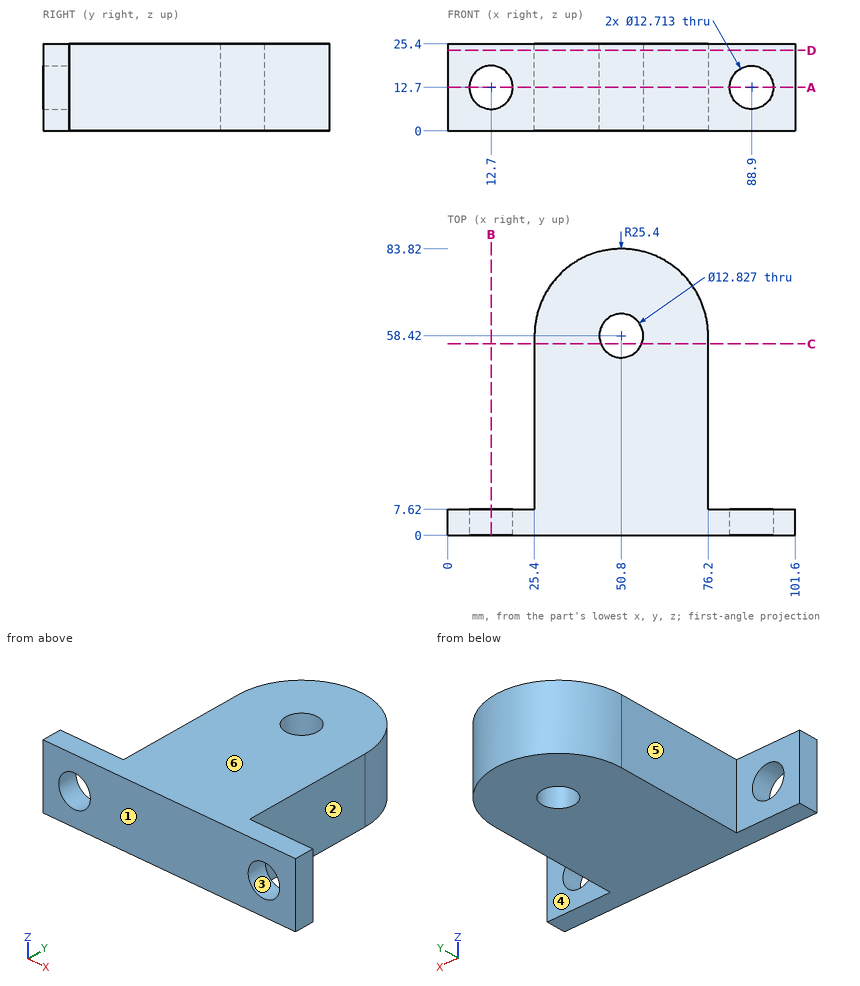
The drawing under review shows one solid part. Ordinate dimensions are in mm from its lowest x, y, z. A direction names the side the tool comes from. Coordinates: 2 decimals unless noted, no trailing zeros. Loops run counter-clockwise (first coordinate to the right, second up) from the corner with the lowest first, then second, coordinate; pieces in that order, holes last. Notation, with made-up numbers: (-33.5, -21.75) - (5.5, -21.75) arc R25 cw to (5.5, -8.75) - close; hole circle Ø7 at (61.5, 43.25). An arc over 180 degrees is marked (long way). Return JSON: item names as keys, results as strings.
Item 1: Take a section at C-C (y = 56). Give the boundary of the cut face in (x, z).
Determined:
{"outline": "(25.4, 0) - (44.86, 0) - (44.86, 25.4) - (25.4, 25.4) - close; (56.74, 0) - (76.2, 0) - (76.2, 25.4) - (56.74, 25.4) - close"}
Item 2: For line 1 (Y direction, x = 50.8, z = 6.75); line 2 (Z direction, x = 88.9, y = 5.5); line 3 (X direction, y = 11.5, z = 10.25), list the stretches that pass through material, from the lowest coordinate up.
Determined:
{"line 1": "y = 0 to 52.01, 64.83 to 83.82", "line 2": "z = 0 to 6.34, 19.06 to 25.4", "line 3": "x = 25.4 to 76.2"}
Item 3: Insertion check: pin 1 (2 mm diameter, centred on y = 71.5, z = 9, fed in from +X); pin 2 (1 mm diameter, centred on y = 74.5, z = 15.5, fed in from -X); pin 3 (16.5 mm diameter, centred on x = 50.8, y = 58.42, fed in from -Z); pin 4 (7.5 mm diameter, centred on x = 92.5, z = 6.5, fed in from +Y). Each pin has a flat end and moves straight along its axis. Give the tip position at first contact, or say it passes through.
Determined:
{"pin 1": "stops at x = 73.14", "pin 2": "stops at x = 30.74", "pin 3": "stops at z = 0", "pin 4": "stops at y = 7.62"}
Item 4: For the marked faces 4, 5 and 6, list the 3-axis set-ups (+Z, -Z, +X, -X, +Y, -Y) from which the entire face can be reached by the end or side of a thin tool; tool diameter is ignored.
Determined:
{"face 4": "+Z, -Z, +X, +Y", "face 5": "+Z, -Z, -X, +Y", "face 6": "+Z, +X, -X, +Y, -Y"}
Item 5: Take a section at B-B (x = 12.7). Give the boundary of the cut face in (y, z).
Determined:
{"outline": "(0, 0) - (7.62, 0) - (7.62, 6.34) - (0, 6.34) - close; (0, 19.06) - (7.62, 19.06) - (7.62, 25.4) - (0, 25.4) - close"}
Item 6: Take a section at A-A (z = 12.7). Give the boundary of the cut face in (x, y), then the cut area to 3 significant figures.
Determined:
{"outline": "(0, 0) - (6.34, 0) - (6.34, 7.62) - (0, 7.62) - close; (19.06, 0) - (82.54, 0) - (82.54, 7.62) - (76.2, 7.62) - (76.2, 58.42) arc R25.4 ccw to (25.4, 58.42) - (25.4, 7.62) - (19.06, 7.62) - close; (95.26, 0) - (101.6, 0) - (101.6, 7.62) - (95.26, 7.62) - close; hole circle Ø12.83 at (50.8, 58.42)", "area": "4,050 mm2"}
Item 7: Take a section at D-D (z = 23.5). Give the boundary of the cut face in (x, y), then the cut area to 3 significant figures.
Determined:
{"outline": "(0, 0) - (101.6, 0) - (101.6, 7.62) - (76.2, 7.62) - (76.2, 58.42) arc R25.4 ccw to (25.4, 58.42) - (25.4, 7.62) - (0, 7.62) - close; hole circle Ø12.83 at (50.8, 58.42)", "area": "4,240 mm2"}
Item 8: Mouldability with a two-part tool opening along X and no side actions: class the marked faces 1, 2 and 3 as pulls with the +X half, pulls with the -X half, needs draft (parallel to the pull), parting line crosses it, or undercut.
Determined:
{"face 1": "needs draft", "face 2": "pulls with the +X half", "face 3": "undercut"}
